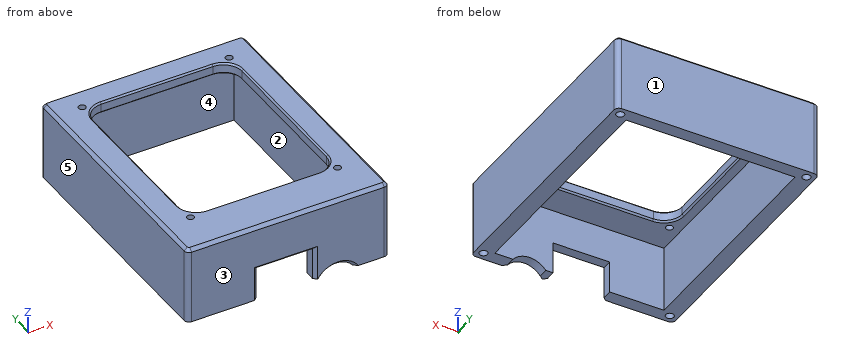
```python
from build123d import *

# Parameters (mm, degrees)
SKETCH1_R           = 1.1
BOSS_EXTRUDE1_DEPTH = 3.5
BOSS_EXTRUDE2_START = 20.759
SKETCH2_R           = 1.25
SKETCH2_W           = 53
SKETCH2_H           = 71.3
BOSS_EXTRUDE2_DEPTH = 20.759
SKETCH3_R           = 6.499999954
SKETCH3_W           = 17.713
SKETCH3_H           = 10
CUT_EXTRUDE1_DEPTH  = 10
CHAMFER1_SIZE       = 1
CHAMFER2_SIZE       = 0.5
CHAMFER3_SIZE       = 1


with BuildPart() as part:
    # Sketch1 → Boss-Extrude1 (new body)
    with BuildSketch(Plane.XY):
        with BuildLine():
            Line((-8.645, -11.5), (-8.645, 64.8))
            ThreePointArc((-8.645, 64.8), (-8.205660172, 65.860660172), (-7.145, 66.3))
            Line((-7.145, 66.3), (53.195, 66.3))
            ThreePointArc((53.195, 66.3), (54.255660172, 65.860660172), (54.695, 64.8))
            Line((54.695, 64.8), (54.695, -11.5))
            ThreePointArc((54.695, -11.5), (54.255660172, -12.560660172), (53.195, -13))
            Line((53.195, -13), (-7.145, -13))
            ThreePointArc((-7.145, -13), (-8.205660172, -12.560660172), (-8.645, -11.5))
        make_face()
        Circle(SKETCH1_R, mode=Mode.SUBTRACT)
        with Locations((0, 58.9)):
            Circle(SKETCH1_R, mode=Mode.SUBTRACT)
        with Locations((46.05, 58.9)):
            Circle(SKETCH1_R, mode=Mode.SUBTRACT)
        with Locations((46.05, 0)):
            Circle(SKETCH1_R, mode=Mode.SUBTRACT)
        with BuildLine():
            Line((5.51, 0.775), (40.54, 0.775))
            ThreePointArc((40.54, 0.775), (44.605863992, 2.459136008), (46.29, 6.525))
            Line((46.29, 6.525), (46.29, 52.375))
            ThreePointArc((46.29, 52.375), (44.605863992, 56.440863992), (40.54, 58.125))
            Line((40.54, 58.125), (5.51, 58.125))
            ThreePointArc((5.51, 58.125), (1.444136008, 56.440863992), (-0.24, 52.375))
            Line((-0.24, 52.375), (-0.24, 6.525))
            ThreePointArc((-0.24, 6.525), (1.444136008, 2.459136008), (5.51, 0.775))
        make_face(mode=Mode.SUBTRACT)
    extrude(amount=BOSS_EXTRUDE1_DEPTH)

    # Sketch2 → Boss-Extrude2 (add)
    with BuildSketch(Plane(origin=(0, 0, 0), x_dir=(-1, 0, 0), z_dir=(0, 0, -1)).offset(BOSS_EXTRUDE2_START)):
        with BuildLine():
            Line((-54.695, -11.5), (-54.695, 64.8))
            ThreePointArc((-54.695, 64.8), (-54.255660172, 65.860660172), (-53.195, 66.3))
            Line((-53.195, 66.3), (7.145, 66.3))
            ThreePointArc((7.145, 66.3), (8.205660172, 65.860660172), (8.645, 64.8))
            Line((8.645, 64.8), (8.645, -11.5))
            ThreePointArc((8.645, -11.5), (8.205660172, -12.560660172), (7.145, -13))
            Line((7.145, -13), (-53.195, -13))
            ThreePointArc((-53.195, -13), (-54.255660172, -12.560660172), (-54.695, -11.5))
        make_face()
        with Locations((-52.195, -10.5)):
            Circle(SKETCH2_R, mode=Mode.SUBTRACT)
        with Locations((6.145, -10.5)):
            Circle(SKETCH2_R, mode=Mode.SUBTRACT)
        with Locations((6.145, 63.8)):
            Circle(SKETCH2_R, mode=Mode.SUBTRACT)
        with Locations((-52.195, 63.8)):
            Circle(SKETCH2_R, mode=Mode.SUBTRACT)
        with Locations((-23.025, 26.65)):
            Rectangle(SKETCH2_W, SKETCH2_H, mode=Mode.SUBTRACT)
    extrude(amount=-BOSS_EXTRUDE2_DEPTH)

    # Sketch3 → Cut-Extrude1 (cut)
    with BuildSketch(Plane.XZ.offset(13)):
        with Locations((38.695, -24.759)):
            Circle(SKETCH3_R)
        with Locations((22.424100803, -15.759)):
            Rectangle(SKETCH3_W, SKETCH3_H)
    extrude(amount=-CUT_EXTRUDE1_DEPTH, mode=Mode.SUBTRACT)

    # Chamfer1
    chamfer1_edges = [part.edges().sort_by_distance(p)[0] for p in [
        (54.255660172, -12.560660172, 3.5),
        (54.695, 26.65, 3.5),
        (54.255660172, 65.860660172, 3.5),
        (23.025, 66.3, 3.5),
        (-8.205660172, 65.860660172, 3.5),
        (-8.645, 26.65, 3.5),
        (-8.205660172, -12.560660172, 3.5),
        (23.025, -13, 3.5),
    ]]
    chamfer(chamfer1_edges, length=CHAMFER1_SIZE)

    # Chamfer2
    chamfer2_edges = [part.edges().sort_by_distance(p)[0] for p in [
        (44.605863992, 2.459136008, 0),
        (46.29, 29.45, 0),
        (44.605863992, 56.440863992, 0),
        (23.025, 58.125, 0),
        (1.444136008, 56.440863992, 0),
        (-0.24, 29.45, 0),
        (1.444136008, 2.459136008, 0),
        (23.025, 0.775, 0),
        (44.605863992, 2.459136008, 3.5),
        (46.29, 29.45, 3.5),
        (44.605863992, 56.440863992, 3.5),
        (23.025, 58.125, 3.5),
        (1.444136008, 56.440863992, 3.5),
        (-0.24, 29.45, 3.5),
        (1.444136008, 2.459136008, 3.5),
        (23.025, 0.775, 3.5),
    ]]
    chamfer(chamfer2_edges, length=CHAMFER2_SIZE)

    # Chamfer3
    chamfer3_edges = [part.edges().sort_by_distance(p)[0] for p in [
        (38.695, -13, -18.259000046),
        (13.567600803, -13, -15.759),
        (31.280600803, -13, -15.759),
        (22.424100803, -13, -10.759),
    ]]
    chamfer(chamfer3_edges, length=CHAMFER3_SIZE)


solid = part.part
```
Check sheet for the modelled part. Datum: model origin and axes. Units: mm. Face numbers are marked on the shaded views. A direction names the side the tool comes from. Give positions to 0.01 mm unless a question says otherwise; leave off trailing zeros. Loops run counter-clockwise (first coordinate to the right, second up) from the corner with the lowest first, then second, coordinate; pieces in that order, holes last. Notation, with made-up numbers: M 43,85.25 L 78,85.25 A24 cw 78,111.25 Z; hole C 78.25,47.5 d4. An arc over 180 degrees is marked long. Answer in a Markdown table with one row per item.
1) Thickness scan on line 1 (X direction, y = 46, z = -17) (3 decimals); line 2 (Y direction, x = 29.5, z = 0.5) (3 decimals); line 3 (Y direction, x = 42, z = -14.75). Record the ranges inside material, lowest first.
Solutions:
| item | result |
|---|---|
| line 1 | x = -8.645 to -3.475, 49.525 to 54.695 |
| line 2 | y = -13 to 0.775, 58.125 to 66.3 |
| line 3 | y = -13 to -9, 62.3 to 66.3 |
2) Cross-section at B-B (y = 36.5). Enter the section's corners in (x, z) (3 decimals), plus the area to 3 significant figures.
Solutions:
| item | result |
|---|---|
| outline | M -8.645,-20.759 L -3.475,-20.759 L -3.475,0 L -0.74,0 L -0.24,0.5 L -0.24,3 L -0.74,3.5 L -7.645,3.5 L -8.645,2.5 Z; M 46.29,0.5 L 46.79,0 L 49.525,0 L 49.525,-20.759 L 54.695,-20.759 L 54.695,2.5 L 53.695,3.5 L 46.79,3.5 L 46.29,3 Z |
| area | 272 mm^2 |
3) Tool access check on the marked faces 4 and 5. Record the directions out of +Z, -Z, +X, -X, +Y, -Y that give a thin tool (end or side, any length) a straight path to the whole face; none if there is none.
Solutions:
| item | result |
|---|---|
| face 4 | -Z |
| face 5 | +Z, -Z, -X, +Y, -Y |
4) Mould release check, pull along Y, two halves, no side actions. Record for the marked faces 1, 2 and 3: released by +Y, released by -Y, zero draft, split by the parting line, or undercut.
Solutions:
| item | result |
|---|---|
| face 1 | released by +Y |
| face 2 | undercut |
| face 3 | released by -Y |
5) Cross-section at A-A (z = -14.5). Enter the section's corners in (x, y) (3 decimals).
Solutions:
| item | result |
|---|---|
| outline | M -8.645,-11.5 A1.5 ccw -7.145,-13 L 12.568,-13 L 13.568,-12 L 13.568,-9 L -3.475,-9 L -3.475,62.3 L 49.525,62.3 L 49.525,-9 L 31.281,-9 L 31.281,-12 L 32.281,-13 L 53.195,-13 A1.5 ccw 54.695,-11.5 L 54.695,64.8 A1.5 ccw 53.195,66.3 L -7.145,66.3 A1.5 ccw -8.645,64.8 Z; hole C -6.145,-10.5 d2.5; hole C -6.145,63.8 d2.5; hole C 52.195,-10.5 d2.5; hole C 52.195,63.8 d2.5 |
6) Depth check by flat-ended pin: pin 1 (4 mm diameter, centred on x = -2, y = 41, fed in from -Z); pin 2 (2 mm diameter, centred on x = 0, y = 0, fed in from -Z) (3 decimals); pin 3 (1.5 mm diameter, centred on x = 18.5, y = -11, fed in from -Z); pin 4 (1.2 mm diameter, centred on x = -6.5, y = -11, fed in from -Z). Enter the tip coordinate at first touch or a pass-through.
Solutions:
| item | result |
|---|---|
| pin 1 | stops at z = -20.76 |
| pin 2 | passes through |
| pin 3 | stops at z = -10.76 |
| pin 4 | stops at z = 0 |
7) Cross-section at D-D (y = 63.8). Enter the section's corners in (x, z) (3 decimals), plus the area to 3 significant figures.
Solutions:
| item | result |
|---|---|
| outline | M -8.645,-20.759 L -7.395,-20.759 L -7.395,0 L -4.895,0 L -4.895,-20.759 L 50.945,-20.759 L 50.945,0 L 53.445,0 L 53.445,-20.759 L 54.695,-20.759 L 54.695,2.5 L 53.695,3.5 L -7.645,3.5 L -8.645,2.5 Z |
| area | 1,430 mm^2 |
8) Cross-section at C-C (x = 10). Enter the section's corners in (y, z) (3 decimals), plus the area to 3 significant figures.
Solutions:
| item | result |
|---|---|
| outline | M -13,-20.759 L -9,-20.759 L -9,0 L 0.275,0 L 0.775,0.5 L 0.775,3 L 0.275,3.5 L -12,3.5 L -13,2.5 Z; M 58.125,0.5 L 58.625,0 L 62.3,0 L 62.3,-20.759 L 66.3,-20.759 L 66.3,2.5 L 65.3,3.5 L 58.625,3.5 L 58.125,3 Z |
| area | 241 mm^2 |
